from build123d import *

# Parameters (mm, degrees)
SKETCH1_W           = 90
SKETCH1_H           = 58
BOSS_EXTRUDE1_DEPTH = 22
SKETCH2_W           = 90
SKETCH2_H           = 27
CUT_EXTRUDE1_DEPTH  = 24
CUT_EXTRUDE2_DEPTH  = 86.586213843
CUT_EXTRUDE3_REACH  = 78.636
SKETCH4_W           = 24
SKETCH4_H           = 10


with BuildPart() as part:
    # Sketch1 → Boss-Extrude1 (new, symmetric)
    with BuildSketch(Plane.XY):
        with Locations((0, 29)):
            Rectangle(SKETCH1_W, SKETCH1_H)
    extrude(amount=BOSS_EXTRUDE1_DEPTH, both=True)

    # Sketch2 → Cut-Extrude1 (cut)
    with BuildSketch(Plane.XY.offset(22)):
        with Locations((0, 31.5)):
            Rectangle(SKETCH2_W, SKETCH2_H)
    extrude(amount=-CUT_EXTRUDE1_DEPTH, mode=Mode.SUBTRACT)

    # Sketch3 → Cut-Extrude2 (cut, through all)
    with BuildSketch(Plane(origin=(0, 0, -22), x_dir=(-1, 0, 0), z_dir=(0, 0, -1))):
        Polygon((-45, 58), (-45, 0), (-22, 58), align=None)
    cut_extrude2 = extrude(amount=-CUT_EXTRUDE2_DEPTH, mode=Mode.SUBTRACT)

    # Mirror1: Cut-Extrude2 across plane
    add(cut_extrude2.mirror(Plane(origin=(0, 0, 0), x_dir=(0, 0, 1), z_dir=(1, 0, 0))), mode=Mode.SUBTRACT)

    # Sketch4 → Cut-Extrude3 (cut, up to next)
    with BuildSketch(Plane.XZ, mode=Mode.PRIVATE) as cut_extrude3_sk1:
        with Locations((0, 17)):
            Rectangle(SKETCH4_W, SKETCH4_H)
    cut_extrude3_tool1 = extrude(cut_extrude3_sk1.sketch, amount=-CUT_EXTRUDE3_REACH, mode=Mode.PRIVATE) & part.part
    add(cut_extrude3_tool1.solids().sort_by_distance((0, 0, 17))[0], mode=Mode.SUBTRACT)


solid = part.part
The model under review builds one solid part; all positions refer to its coordinate system, in mm. A direction names the side the tool comes from. Round coordinates to 2 decimals unless told otherwise and drop trailing zeros. Loops run counter-clockwise (first coordinate to the right, second up) from the corner with the lowest first, then second, coordinate; pieces in that order, holes last. Notation, with made-up numbers: (18.5, -28) -> (35.5, -28) arc R22 cw to (35.5, -15) -> close; hole circle Ø8 at (50.25, 71). An arc over 180 degrees is marked (long way). One line per question, with ' | ' between items. Start each with the question number.
Item 1: Draft analysis for pull direction Y (two halves, no side actions). For faces 1 (the face through (0, 58, 0)), 2 (the face through (-1, 32, -2)), 3 (the face through (28, 9, 22)), state which applies: +Y half, -Y half, draft (parallel to the pull), parting line (faces both ways), or undercut.
Item 2: Add section C-C, the plane x = 5.5. Write out the cut boundary in (y, z), then the cut area to 3 significant figures.
Item 3: Add section D-D, the plane y = 8.5. Write out the cut boundary in (x, z).
Item 4: Wall thickness on line 1 along Y through (x, z) = (21, -1); line 2 along Z through (x, y) = (-33, 28); line 3 along Y through (x, z) = (-28, 7.5): over which ranges is each line inside the solid? List them lowest first. Write a range as [from, to].
Item 5: Add section A-A, the plane z = 5.5. Write out the cut boundary in (x, y), then the cut area to 3 significant figures.
Item 6: For pin 1 (5 mm diameter, centred on y = 5.5, z = 14.5, fed in from -X); pin 2 (5.5 mm diameter, centred on x = -3, y = 6, fed in from +Z); pin 3 (5 mm diameter, centred on y = 7, z = 14.5, fed in from +X), all flat-tipped, find the tip position at first contact; note any pin that passes through.
Item 7: Add section B-B, the plane z = 19. Write out the cut boundary in (x, y), then the cut area to 3 significant figures.
Item 8: Machinability: for faces 4 (the face through (-29, 9, 22)), 5 (the face through (-12, 9, 17)), 6 (the face through (-1, 18, 10)), which of the approach directions +Z, -Z, +X, -X, +Y, -Y give a long, thin tool a straight path to every point of the face, cutting with its end or side? Answer none if there is none.
Return value:
1) face 1: +Y half | face 2: undercut | face 3: draft
2) outline: (0, -22) -> (58, -22) -> (58, 22) -> (45, 22) -> (45, -2) -> (18, -2) -> (18, 12) -> (0, 12) -> close | area: 1,720 mm2
3) outline: (-41.63, -22) -> (41.63, -22) -> (41.63, 22) -> (12, 22) -> (12, 12) -> (-12, 12) -> (-12, 22) -> (-41.63, 22) -> close
4) line 1: y = [0, 18], [45, 58] | line 2: z = [-22, -2] | line 3: y = [0, 18]
5) outline: (-45, 0) -> (45, 0) -> (37.86, 18) -> (-37.86, 18) -> close; (-27.16, 45) -> (27.16, 45) -> (22, 58) -> (-22, 58) -> close | area: 2,130 mm2
6) pin 1: stops at x = -43.81 | pin 2: stops at z = 12 | pin 3: stops at x = 43.22
7) outline: (-45, 0) -> (-12, 0) -> (-12, 18) -> (-37.86, 18) -> close; (-27.16, 45) -> (27.16, 45) -> (22, 58) -> (-22, 58) -> close; (12, 0) -> (45, 0) -> (37.86, 18) -> (12, 18) -> close | area: 1,700 mm2
8) face 4: +Z, +X, -X, +Y, -Y | face 5: +Z, -Y | face 6: +Z, +X, -X
